Geometry check sheet. Reference: the model listing, model coordinates, mm. A direction names the side the tool comes from. Coordinates: 2 decimals unless noted, no trailing zeros. Write each loop counter-clockwise with the first axis right and the second up, starting at its lowest first coordinate (ties: lowest second). Pieces come first, ordered by that corner, then holes. Notation, with made-up numbers: M 0,12.25 L 41,12.25 A24 ccw 41,32.25 Z; hole C -30,64.5 d7. An arc over 180 degrees is marked long. Write item = value, one per line. Start each with the question number.
```python
from build123d import *

# Parameters (mm, degrees)
CROQUIS1_R                 = 7.9375
SALIENTE_EXTRUIR1_DEPTH    = 200
CORTAR_EXTRUIR1_DEPTH      = 16.565810413
CORTAR_EXTRUIR1_DEPTH_BACK = 201.314771828
CROQUIS2_R                 = 1.5875
CORTAR_EXTRUIR2_DEPTH      = 201.314771936
CORTAR_EXTRUIR2_DEPTH_BACK = 16.77901512
CROQUIS3_R                 = 3.175
CROQUIS4_W                 = 20
CROQUIS4_H                 = 19.524905572
CROQUIS4_H_2               = 20.597317053
CROQUIS4_W_2               = 30
CROQUIS4_H_3               = 3.175
CORTAR_EXTRUIR3_DEPTH      = 2
CROQUIS5_W                 = 4
CROQUIS5_H                 = 10.535653752
SALIENTE_EXTRUIR2_DEPTH    = 30
CROQUIS6_R                 = 3
CORTAR_EXTRUIR4_DEPTH      = 232


with BuildPart() as part:
    # Croquis1 → Saliente-Extruir1 (new, symmetric)
    with BuildSketch(Plane.XY):
        Circle(CROQUIS1_R)
    extrude(amount=SALIENTE_EXTRUIR1_DEPTH, both=True)

    # Croquis2 → Cortar-Extruir1 (cut, two sides: drawn at the far end of the back side and taken through both)
    with BuildSketch(Plane(origin=(0, 0, 0), x_dir=(0, 0, -1), z_dir=(1, 0, 0)).offset(-CORTAR_EXTRUIR1_DEPTH_BACK)):
        with Locations(Location((194, 0, 0), (0, 0, 180))):
            Circle(CROQUIS2_R)
    extrude(amount=CORTAR_EXTRUIR1_DEPTH + CORTAR_EXTRUIR1_DEPTH_BACK, mode=Mode.SUBTRACT)

    # Croquis3 → Cortar-Extruir2 (cut, two sides: drawn at the far end of the back side and taken through both)
    with BuildSketch(Plane(origin=(0, 0, 0), x_dir=(1, 0, 0), z_dir=(0, 1, 0)).offset(-CORTAR_EXTRUIR2_DEPTH_BACK)):
        with Locations(Location((0, -193.067059354, 0), (0, 0, 270))):
            Circle(CROQUIS3_R)
    extrude(amount=CORTAR_EXTRUIR2_DEPTH + CORTAR_EXTRUIR2_DEPTH_BACK, mode=Mode.SUBTRACT)

    # Croquis4 → Cortar-Extruir3 (cut)
    with BuildSketch(Plane(origin=(7.9375, 0, 0), x_dir=(0, 0, -1), z_dir=(1, 0, 0))):
        with Locations((71.2, -0.983446493)):
            Rectangle(CROQUIS4_W, CROQUIS4_H)
        with Locations((-53.151122479, -1.451804467)):
            Rectangle(CROQUIS4_W, CROQUIS4_H_2)
        with Locations((-167.851453134, -1.451804466)):
            Rectangle(CROQUIS4_W_2, CROQUIS4_H_3)
    extrude(amount=-CORTAR_EXTRUIR3_DEPTH, mode=Mode.SUBTRACT)

    # Croquis5 → Saliente-Extruir2 (add)
    with BuildSketch(Plane(origin=(5.9375, 0, 0), x_dir=(0, 0, -1), z_dir=(1, 0, 0))):
        with Locations((66.325, 0)):
            Rectangle(CROQUIS5_W, CROQUIS5_H)
        with Locations((76.075, 0)):
            Rectangle(CROQUIS5_W, CROQUIS5_H)
        with Locations((-49.713622479, 0)):
            Rectangle(CROQUIS5_W, CROQUIS5_H)
        with Locations((-58.026122479, 0)):
            Rectangle(CROQUIS5_W, CROQUIS5_H)
    extrude(amount=SALIENTE_EXTRUIR2_DEPTH)

    # Croquis6 → Cortar-Extruir4 (cut)
    with BuildSketch(Plane(origin=(0, 0, -78.075), x_dir=(-1, 0, 0), z_dir=(0, 0, -1))):
        with Locations((-29.9375, 0)):
            Circle(CROQUIS6_R)
    extrude(amount=-CORTAR_EXTRUIR4_DEPTH, mode=Mode.SUBTRACT)


solid = part.part
```
Q1. Cross-section at A-A on x = 14. Enter the section's corners in (y, z) (3 decimals), and give its area (3 significant figures).
Q2. Cross-section at B-B on z = -33. Enter the section's corners in (x, y) (1 decimal), and give its area (3 significant figures).
Q3. Scan lines: L1, parallel to Z at x = 31, y = -5 (3 decimals); L2, parallel to Z at x = 2, y = 0.75; L3, parallel to Y at x = 1.25, z = -194. Record each from-to range of solid material in increasing order.
Q4. Draft check along Z on faces 1 (the face through (21, 0, -64.325)), 2 (the face through (0, 0, 200)), 3 (the face through (0, 0, -200)), 4 (the face through (21, 0, -68.325)). Enter one of: pulls with the +Z half, pulls with the -Z half, needs draft (parallel to the pull), parting line crosses it, or undercut.
Q5. Set-up check for faces 5 (the face through (-1.22, -0.11, 196)), 6 (the face through (21, 0, -74.075)), 7 (the face through (-7.93, 0.35, 2.8)): record each of +Z, -Z, +X, -X, +Y, -Y from which the full face is reachable in a straight line by a thin tool's end or side.
Q6. Gauge pin test, flat ends, axial feed: pin 1 (2.5 mm diameter, centred on y = 1, z = 45, fed in from +X); pin 2 (1.5 mm diameter, centred on y = 3, z = -39.5, fed in from -X); pin 3 (1.2 mm diameter, centred on x = 22.5, z = -67, fed in from -Y); pin 4 (3.5 mm diameter, centred on x = 29.94, y = 0, fed in from +Z). Record the tip position at first contact, or that the pin passes through.
Values found:
q1.outline = M -5.268,-78.075 L 5.268,-78.075 L 5.268,-74.075 L -5.268,-74.075 Z; M -5.268,-68.325 L 5.268,-68.325 L 5.268,-64.325 L -5.268,-64.325 Z; M -5.268,47.714 L 5.268,47.714 L 5.268,51.714 L -5.268,51.714 Z; M -5.268,56.026 L 5.268,56.026 L 5.268,60.026 L -5.268,60.026 Z
q1.area = 169 mm²
q2.outline = C 0,0 d15.9
q2.area = 198 mm²
q3.L1 = -78.075 to -74.075, -68.325 to -64.325, 47.714 to 51.714, 56.026 to 60.026
q3.L2 = -200 to -195.4, -192.6 to 190.6, 195.53 to 200
q3.L3 = -7.84 to -1.59, 1.59 to 7.84
q4.face_1 = undercut
q4.face_2 = pulls with the +Z half
q4.face_3 = pulls with the -Z half
q4.face_4 = undercut
q5.face_5 = +Y, -Y
q5.face_6 = +X, +Y, -Y
q5.face_7 = none
q6.pin_1 = 5.94
q6.pin_2 = -7.61
q6.pin_3 = -5.27
q6.pin_4 = through
